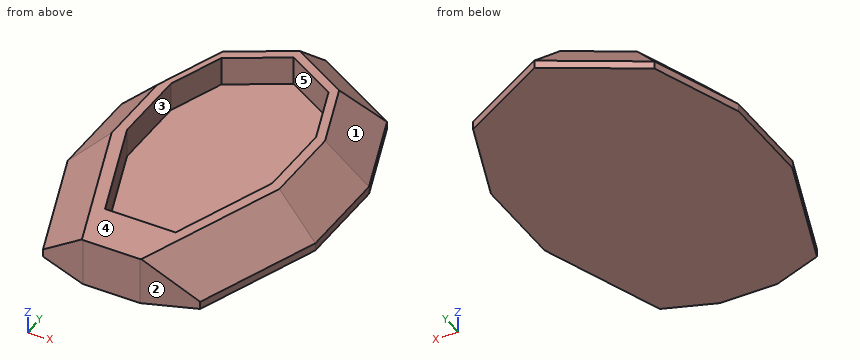
```python
from build123d import *

# Parameters (mm, degrees)
F1_DEPTH = 10
F2_DEPTH = 90
F3_SIZE2 = 83.771
F3_SIZE  = 83.771
F5_DEPTH = 60


# Not quite as in the source:
# - a feature names something its author has since deleted; it is built from what else it names


with BuildPart() as f1:
    # F0 (on Top) → F1 (new body)
    with BuildSketch(Plane.XY):
        Polygon((190.5255888326, 290), (0, 400), (-190.5255888326, 290), (-260, 99.1206240876), (-260, -100.8793759124), (-165.0447262585, -361.7668463753), (-60, -400), (60, -400), (165.0447262585, -361.7668463753), (260, -100.8793759124), (260, 99.1206240876), align=None)
    extrude(amount=F1_DEPTH)

    # F2 (add): a face of the model
    f2_faces = [f1.faces().sort_by_distance(p)[0] for p in [
        (0, -14.4086757736, 10),
    ]]
    extrude(f2_faces, amount=F2_DEPTH)

    # F3
    f3_edges = [f1.edges().sort_by_distance(p)[0] for p in [
        (-212.522363, -231.323111, 100),
        (212.522363, -231.323111, 100),
        (260, -0.879376, 100),
        (225.262794, 194.560312, 100),
        (95.262794, 345, 100),
        (-95.262794, 345, 100),
        (-225.262794, 194.560312, 100),
        (-260, -0.879376, 100),
    ]]
    chamfer(f3_edges, length=F3_SIZE, length2=F3_SIZE2)

    # F4 (on face) → F5 (cut)
    with BuildSketch(Plane.XY.offset(100)):
        Polygon((-114.5740551886, 214.0262088265), (-156.229, 99.5801885487), (-156.229, -63.8245572211), (-71.6236926582, -296.2757287087), (76.4689935111, -296.2757287087), (156.229, -77.136911905), (156.229, 86.2678338648), (108.4396889686, 217.567886815), (0, 280.1755704318), align=None)
    extrude(amount=-F5_DEPTH, mode=Mode.SUBTRACT)


solid = f1.part
```
Geometry: final body of the model. Coordinates: model frame, mm. Face numbers are marked on the shaded views. A direction names the side the tool comes from. Give positions to 0.01 mm unless a question says otherwise; leave off trailing zeros. Write each loop counter-clockwise with the first axis right and the second up, starting at its lowest first coordinate (ties: lowest second). Pieces come first, ordered by that corner, then holes.
1. Draft query along Y for the marked faces 1, 2 and 3. Return one class per face: released by +Y, released by -Y, zero draft, split by the parting line, or undercut.
2. Pin query (flat end, axial travel): P1, Ø4, axis at x = 167, z = 45.5, coming from the +Y side; P2, Ø12, axis at x = 133, z = 19, coming from the -Y side; P3, Ø6, axis at y = 28, z = 63.5, coming from the -X side. Return the tip coordinate at first contact, or that it passes through.
3. Section query D-D, the plane y = 317. Return loops of the section in (x, z), then the cut area to 3 significant figures.
4. Section query B-B, the plane y = -212. Return loops of the section in (x, z).
5. Reachability of the marked faces 4 and 5 from +Z, -Z, +X, -X, +Y, -Y: full face, straight path, thin tool, end or side. Return the list, or none.
6. Line query: probe 1 along X at (y, z) = (138.5, 60); probe 2 along X at (y, z) = (-122, 59.5); probe 3 along Z at (x, y) = (136, -104). Output: solid intervals per line, ascending.
7. Section query A-A, the plane z = 84. Return loops of the section in (x, y).
8. Section query C-C, the plane x = -16. Return loops of the section in (y, z), then the cut area to 3 significant figures.
Computed:
1. face 1: released by +Y
1. face 2: released by -Y
1. face 3: undercut
2. P1: stops at y = 272.37
2. P2: stops at y = -375.61
2. P3: stops at x = -215.73
3. outline: (-143.76, 0) - (143.76, 0) - (143.76, 16.23) - (0, 88.11) - (-143.76, 16.23) - close
3. area: 15,000 mm2
4. outline: (-219.56, 0) - (219.56, 0) - (219.56, 16.23) - (130.41, 100) - (107.14, 100) - (107.14, 40) - (-102.3, 40) - (-102.3, 100) - (-130.41, 100) - (-219.56, 16.23) - close
5. face 4: +Z, +X, -X, +Y, -Y
5. face 5: +Z
6. probe 1: x = -199.09 to -142.06, 137.22 to 199.09
6. probe 2: x = -206.26 to -135.05, 139.9 to 206.26
6. probe 3: z = 0 to 40
7. outline: (-192.23, -88.93) - (-81.91, -392.02) - (-60, -400) - (60, -400) - (81.91, -392.02) - (192.23, -88.93) - (192.23, 87.17) - (135.28, 243.64) - (0, 321.74) - (-135.28, 243.64) - (-192.23, 87.17) - close; hole (-156.23, -63.82) - (-71.62, -296.28) - (76.47, -296.28) - (156.23, -77.14) - (156.23, 86.27) - (108.44, 217.57) - (0, 280.18) - (-114.57, 214.03) - (-156.23, 99.58) - close
8. outline: (-400, 0) - (390.76, 0) - (390.76, 16.23) - (294.03, 100) - (270.94, 100) - (270.94, 40) - (-296.28, 40) - (-296.28, 100) - (-400, 100) - close
8. area: 41,000 mm2
